Read the model definition and answer for the solid it produces. Units are mm, in the model's axes. A direction names the side the tool comes from. Coordinates: 2 decimals unless noted, no trailing zeros. Order: outer loops, then holes, each group sorted by start corner. A loop starts at its lowest first (then second) coordinate and runs counter-clockwise, first axis right, second up. Notation, with made-up numbers: (13.5, -31.5) -> (46.5, -31.5) arc R14 cw to (46.5, -16.5) -> close; hole circle Ø6 at (38.5, 2). An arc over 180 degrees is marked (long way). Answer as a JSON object with one key per item and string values. Group by question number.
1) A tool of negligible diameter and unlimited length cuts with its end or side. For faces 1 (the flat face through (58.7, 180.5, 8)), 2 (the flat face through (105, 90, 2)), 3 (the flat face through (58.7, 0.5, 8)), 4 (the flat face through (109, 91, 4)), from which of +Z, -Z, +X, -X, +Y, -Y can it reach the whole face along a straight path? Write none if from no direction.
2) Section A-A on x = 31 is taken. Determine the outline of the cut face in (y, z), and give its area (3 significant figures).
3) Given pin 1 (1.8 mm diameter, centred on x = 14.5, y = 183, fed in from -Z); pin 2 (2 mm diameter, centred on x = 62.5, z = 2, fed in from -Y); pin 3 (1.2 mm diameter, centred on y = -1.5, z = 7, fed in from +X), each flat-ended and moving along its own axis, determine where each tip first touches the part or whether it passes through.
4) Consider L1, parallel to Y at x = 26, z = 2.5; L2, parallel to Y at x = 70, z = 7; L3, parallel to X at y = 32.5, z = 9.5. Determine where each line is inside the solid, lowest interval first.
5) Section B-B on y = 167 is taken. Determine the outline of the cut face in (x, z), and give its area (3 significant figures).
6) Determine the mould class of faces 5 (the flat face through (100, -2, 5)), 6 (the flat face through (4, 89, 8)) for opening direction Y: released by +Y, released by -Y, zero draft, split by the parting line, or undercut.
7) Section D-D on y = 101.5 is taken. Determine the outline of the cut face in (x, z), and give its area (4 significant figures).
8) Section C-C on x = 74 is taken. Determine the outline of the cut face in (y, z).
from build123d import *

# Parameters (mm, degrees)
BOX011_W      = 4
BOX011_H      = 80
BOX011_DEPTH  = 3
FILLET006_R   = 1
BOX010_W      = 30
BOX010_H      = 4
BOX010_DEPTH  = 3
FILLET007_R   = 1
BOX009_W      = 30
BOX009_H      = 4
BOX009_DEPTH  = 3
FILLET008_R   = 1
BOX008_W      = 30
BOX008_H      = 4
BOX008_DEPTH  = 3
FILLET009_R   = 1
BOX013_W      = 4
BOX013_H      = 80
BOX013_DEPTH  = 3
FILLET010_R   = 1
BOX012_W      = 30
BOX012_H      = 4
BOX012_DEPTH  = 3
FILLET005_R   = 1
BOX006_W      = 80
BOX006_H      = 10
BOX006_DEPTH  = 10
BOX007_W      = 80
BOX007_H      = 10
BOX007_DEPTH  = 10
FILLET004_1_R = 2
FILLET004_2_R = 1
BOX003_W      = 116
BOX003_H      = 179.5
BOX003_DEPTH  = 10
FILLET002_R   = 1.5
BOX002_W      = 120
BOX002_H      = 181
BOX002_DEPTH  = 8
FILLET003_R   = 1.5
BOX001_W      = 98
BOX001_H      = 173.5
BOX001_DEPTH  = 4
FILLET_R      = 1.5
BOX_W         = 120
BOX_H         = 181
BOX_DEPTH     = 4
FILLET001_R   = 1.5


with BuildPart() as fillet006:
    # Box011 → Box011 (new body)
    with BuildSketch(Plane(origin=(0, 50, 5), x_dir=(1, 0, 0), z_dir=(0, 0, 1))):
        with Locations((2, 40)):
            Rectangle(BOX011_W, BOX011_H)
    extrude(amount=BOX011_DEPTH)

    # Fillet006
    fillet006_edges = [fillet006.edges().sort_by_distance(p)[0] for p in [
        (0, 50, 6.5),
        (0, 130, 6.5),
    ]]
    fillet(fillet006_edges, radius=FILLET006_R)


with BuildPart() as fillet007:
    # Box010 → Box010 (new body)
    with BuildSketch(Plane(origin=(85, -3.5, 5), x_dir=(1, 0, 0), z_dir=(0, 0, 1))):
        with Locations((15, 2)):
            Rectangle(BOX010_W, BOX010_H)
    extrude(amount=BOX010_DEPTH)

    # Fillet007
    fillet007_edges = [fillet007.edges().sort_by_distance(p)[0] for p in [
        (85, -3.5, 6.5),
        (115, -3.5, 6.5),
    ]]
    fillet(fillet007_edges, radius=FILLET007_R)


with BuildPart() as fillet008:
    # Box009 → Box009 (new body)
    with BuildSketch(Plane(origin=(4, 180.5, 5), x_dir=(1, 0, 0), z_dir=(0, 0, 1))):
        with Locations((15, 2)):
            Rectangle(BOX009_W, BOX009_H)
    extrude(amount=BOX009_DEPTH)

    # Fillet008
    fillet008_edges = [fillet008.edges().sort_by_distance(p)[0] for p in [
        (4, 184.5, 6.5),
        (34, 184.5, 6.5),
    ]]
    fillet(fillet008_edges, radius=FILLET008_R)


with BuildPart() as fillet009:
    # Box008 → Box008 (new body)
    with BuildSketch(Plane(origin=(85, 180.5, 5), x_dir=(1, 0, 0), z_dir=(0, 0, 1))):
        with Locations((15, 2)):
            Rectangle(BOX008_W, BOX008_H)
    extrude(amount=BOX008_DEPTH)

    # Fillet009
    fillet009_edges = [fillet009.edges().sort_by_distance(p)[0] for p in [
        (85, 184.5, 6.5),
        (115, 184.5, 6.5),
    ]]
    fillet(fillet009_edges, radius=FILLET009_R)


with BuildPart() as fillet010:
    # Box013 → Box013 (new body)
    with BuildSketch(Plane(origin=(120.5, 50, 5), x_dir=(1, 0, 0), z_dir=(0, 0, 1))):
        with Locations((2, 40)):
            Rectangle(BOX013_W, BOX013_H)
    extrude(amount=BOX013_DEPTH)

    # Fillet010
    fillet010_edges = [fillet010.edges().sort_by_distance(p)[0] for p in [
        (124.5, 50, 6.5),
        (124.5, 130, 6.5),
    ]]
    fillet(fillet010_edges, radius=FILLET010_R)


with BuildPart() as fusion002:
    # Box012 → Box012 (new body)
    with BuildSketch(Plane(origin=(4, -3.5, 5), x_dir=(1, 0, 0), z_dir=(0, 0, 1))):
        with Locations((15, 2)):
            Rectangle(BOX012_W, BOX012_H)
    extrude(amount=BOX012_DEPTH)

    # Fillet005
    fillet005_edges = [fusion002.edges().sort_by_distance(p)[0] for p in [
        (4, -3.5, 6.5),
        (34, -3.5, 6.5),
    ]]
    fillet(fillet005_edges, radius=FILLET005_R)

    # Fusion002: union Fillet006, Fillet007, Fillet008, Fillet009, Fillet010
    add(fillet006.part)
    add(fillet007.part)
    add(fillet008.part)
    add(fillet009.part)
    add(fillet010.part)


with BuildPart() as cube006:
    # Box006 → Box006 (new body)
    with BuildSketch(Plane(origin=(15, -5, 0), x_dir=(1, 0, 0), z_dir=(0, 0, 1))):
        with Locations((40, 5)):
            Rectangle(BOX006_W, BOX006_H)
    extrude(amount=BOX006_DEPTH)


with BuildPart() as fillet004:
    # Box007 → Box007 (new body)
    with BuildSketch(Plane(origin=(15, 175, 0), x_dir=(1, 0, 0), z_dir=(0, 0, 1))):
        with Locations((40, 5)):
            Rectangle(BOX007_W, BOX007_H)
    extrude(amount=BOX007_DEPTH)

    # Fusion: union Cube006
    add(cube006.part)


with BuildPart() as fillet004_1:
    # Fusion placement: moved
    add(fillet004.part.moved(Location((0, 0, 8))))

    # Fillet004 1
    fillet004_1_edges = [fillet004_1.edges().sort_by_distance(p)[0] for p in [
        (15, 180, 8),
        (95, 180, 8),
    ]]
    fillet(fillet004_1_edges, radius=FILLET004_1_R)

    # Fillet004 2
    fillet004_2_edges = [fillet004_1.edges().sort_by_distance(p)[0] for p in [
        (15, 0, 8),
        (95, 0, 8),
    ]]
    fillet(fillet004_2_edges, radius=FILLET004_2_R)


with BuildPart() as fillet002:
    # Box003 → Box003 (new body)
    with BuildSketch(Plane(origin=(4, 0.75, 4), x_dir=(1, 0, 0), z_dir=(0, 0, 1))):
        with Locations((58, 89.75)):
            Rectangle(BOX003_W, BOX003_H)
    extrude(amount=BOX003_DEPTH)

    # Fillet002
    fillet002_edges = [fillet002.edges().sort_by_distance(p)[0] for p in [
        (4, 0.75, 9),
        (4, 180.25, 9),
        (120, 0.75, 9),
        (120, 180.25, 9),
    ]]
    fillet(fillet002_edges, radius=FILLET002_R)


with BuildPart() as cut002:
    # Box002 → Box002 (new body)
    with BuildSketch(Plane(origin=(2, 0, 4), x_dir=(1, 0, 0), z_dir=(0, 0, 1))):
        with Locations((60, 90.5)):
            Rectangle(BOX002_W, BOX002_H)
    extrude(amount=BOX002_DEPTH)

    # Fillet003
    fillet003_edges = [cut002.edges().sort_by_distance(p)[0] for p in [
        (2, 0, 8),
        (2, 181, 8),
        (122, 0, 8),
        (122, 181, 8),
    ]]
    fillet(fillet003_edges, radius=FILLET003_R)

    # Cut001: cut Fillet002
    add(fillet002.part, mode=Mode.SUBTRACT)

    # Cut002: cut Fillet004
    add(fillet004_1.part, mode=Mode.SUBTRACT)


with BuildPart() as fillet_body:
    # Box001 → Box001 (new body)
    with BuildSketch(Plane(origin=(7, 4, 0), x_dir=(1, 0, 0), z_dir=(0, 0, 1))):
        with Locations((49, 86.75)):
            Rectangle(BOX001_W, BOX001_H)
    extrude(amount=BOX001_DEPTH)

    # Fillet
    fillet_edges = [fillet_body.edges().sort_by_distance(p)[0] for p in [
        (7, 4, 2),
        (7, 177.5, 2),
        (105, 4, 2),
        (105, 177.5, 2),
    ]]
    fillet(fillet_edges, radius=FILLET_R)


with BuildPart() as fusion003:
    # Box → Box (new body)
    with BuildSketch(Plane(origin=(2, 0, 0), x_dir=(1, 0, 0), z_dir=(0, 0, 1))):
        with Locations((60, 90.5)):
            Rectangle(BOX_W, BOX_H)
    extrude(amount=BOX_DEPTH)

    # Fillet001
    fillet001_edges = [fusion003.edges().sort_by_distance(p)[0] for p in [
        (2, 0, 2),
        (2, 181, 2),
        (122, 0, 2),
        (122, 181, 2),
    ]]
    fillet(fillet001_edges, radius=FILLET001_R)

    # Cut: cut Fillet body
    add(fillet_body.part, mode=Mode.SUBTRACT)

    # Fusion001: union Cut002
    add(cut002.part)

    # Fusion003: union Fusion002
    add(fusion002.part)


solid = fusion003.part
Worked answers:
{
 "1": {"face 1": "+Z, +Y", "face 2": "+Z, -Z", "face 3": "+Z, -Y", "face 4": "+Z"},
 "2": {"outline": "(-3.5, 5) -> (0, 5) -> (0, 0) -> (4, 0) -> (4, 4) -> (0.75, 4) -> (0.75, 8) -> (-3.5, 8) -> close; (177.5, 0) -> (181, 0) -> (181, 5) -> (184.5, 5) -> (184.5, 8) -> (180.25, 8) -> (180.25, 4) -> (177.5, 4) -> close", "area": "57.0 mm²"},
 "3": {"pin 1": "stops at z = 5", "pin 2": "stops at y = 0", "pin 3": "stops at x = 115"},
 "4": {"L1": "y = 0 to 4, 177.5 to 181", "L2": "y = 0 to 0.75, 180.25 to 181", "L3": "x = 2 to 4, 120 to 122"},
 "5": {"outline": "(2, 0) -> (7, 0) -> (7, 4) -> (4, 4) -> (4, 12) -> (2, 12) -> close; (105, 0) -> (122, 0) -> (122, 12) -> (120, 12) -> (120, 4) -> (105, 4) -> close", "area": "120 mm²"},
 "6": {"face 5": "zero draft", "face 6": "undercut"},
 "7": {"outline": "(0, 5) -> (2, 5) -> (2, 0) -> (7, 0) -> (7, 4) -> (4, 4) -> (4, 12) -> (2, 12) -> (2, 8) -> (0, 8) -> close; (105, 0) -> (122, 0) -> (122, 5) -> (124.5, 5) -> (124.5, 8) -> (122, 8) -> (122, 12) -> (120, 12) -> (120, 4) -> (105, 4) -> close", "area": "133.5 mm²"},
 "8": {"outline": "(0, 0) -> (4, 0) -> (4, 4) -> (0.75, 4) -> (0.75, 8) -> (0, 8) -> close; (177.5, 0) -> (181, 0) -> (181, 8) -> (180.25, 8) -> (180.25, 4) -> (177.5, 4) -> close"}
}
